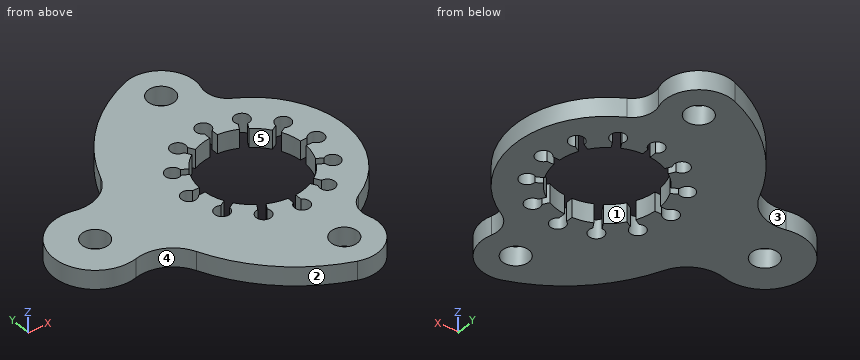
```python
from build123d import *

# Parameters (mm, degrees)
CROQUIS1_R              = 49
CROQUIS1_R_2            = 7
SALIENTE_EXTRUIR1_DEPTH = 10


with BuildPart() as part:
    # Croquis1 → Saliente-Extruir1 (new body)
    # profile 1 of 3: a face of its own
    with BuildSketch(Plane.XY):
        Circle(CROQUIS1_R)
        with BuildLine():
            ThreePointArc((11.73086121, 24.318447633), (6.988114218, 26.07999731), (2, 26.925824036))
            Line((2, 26.925824036), (2, 30.535898385))
            ThreePointArc((2, 30.535898385), (0, 38), (-2, 30.535898385))
            Line((-2, 30.535898385), (-2, 26.925824036))
            ThreePointArc((-2, 26.925824036), (-6.988114218, 26.07999731), (-11.73086121, 24.318447633))
            Line((-11.73086121, 24.318447633), (-13.535898385, 27.444863729))
            ThreePointArc((-13.535898385, 27.444863729), (-19, 32.908965344), (-17, 25.444863729))
            Line((-17, 25.444863729), (-15.194962825, 22.318447633))
            ThreePointArc((-15.194962825, 22.318447633), (-19.091883092, 19.091883092), (-22.318447633, 15.194962825))
            Line((-22.318447633, 15.194962825), (-25.444863729, 17))
            ThreePointArc((-25.444863729, 17), (-32.908965344, 19), (-27.444863729, 13.535898385))
            Line((-27.444863729, 13.535898385), (-24.318447633, 11.73086121))
            ThreePointArc((-24.318447633, 11.73086121), (-26.07999731, 6.988114218), (-26.925824036, 2))
            Line((-26.925824036, 2), (-30.535898385, 2))
            ThreePointArc((-30.535898385, 2), (-38, 0), (-30.535898385, -2))
            Line((-30.535898385, -2), (-26.925824036, -2))
            ThreePointArc((-26.925824036, -2), (-26.07999731, -6.988114218), (-24.318447633, -11.73086121))
            Line((-24.318447633, -11.73086121), (-27.444863729, -13.535898385))
            ThreePointArc((-27.444863729, -13.535898385), (-32.908965344, -19), (-25.444863729, -17))
            Line((-25.444863729, -17), (-22.318447633, -15.194962825))
            ThreePointArc((-22.318447633, -15.194962825), (-19.091883092, -19.091883092), (-15.194962825, -22.318447633))
            Line((-15.194962825, -22.318447633), (-17, -25.444863729))
            ThreePointArc((-17, -25.444863729), (-19, -32.908965344), (-13.535898385, -27.444863729))
            Line((-13.535898385, -27.444863729), (-11.73086121, -24.318447633))
            ThreePointArc((-11.73086121, -24.318447633), (-6.988114218, -26.07999731), (-2, -26.925824036))
            Line((-2, -26.925824036), (-2, -30.535898385))
            ThreePointArc((-2, -30.535898385), (0, -38), (2, -30.535898385))
            Line((2, -30.535898385), (2, -26.925824036))
            ThreePointArc((2, -26.925824036), (6.988114218, -26.07999731), (11.73086121, -24.318447633))
            Line((11.73086121, -24.318447633), (13.535898385, -27.444863729))
            ThreePointArc((13.535898385, -27.444863729), (19, -32.908965344), (17, -25.444863729))
            Line((17, -25.444863729), (15.194962825, -22.318447633))
            ThreePointArc((15.194962825, -22.318447633), (19.091883092, -19.091883092), (22.318447633, -15.194962825))
            Line((22.318447633, -15.194962825), (25.444863729, -17))
            ThreePointArc((25.444863729, -17), (32.908965344, -19), (27.444863729, -13.535898385))
            Line((27.444863729, -13.535898385), (24.318447633, -11.73086121))
            ThreePointArc((24.318447633, -11.73086121), (26.07999731, -6.988114218), (26.925824036, -2))
            Line((26.925824036, -2), (30.535898385, -2))
            ThreePointArc((30.535898385, -2), (38, 0), (30.535898385, 2))
            Line((30.535898385, 2), (26.925824036, 2))
            ThreePointArc((26.925824036, 2), (26.07999731, 6.988114218), (24.318447633, 11.73086121))
            Line((24.318447633, 11.73086121), (27.444863729, 13.535898385))
            ThreePointArc((27.444863729, 13.535898385), (32.908965344, 19), (25.444863729, 17))
            Line((25.444863729, 17), (22.318447633, 15.194962825))
            ThreePointArc((22.318447633, 15.194962825), (19.091883092, 19.091883092), (15.194962825, 22.318447633))
            Line((15.194962825, 22.318447633), (17, 25.444863729))
            ThreePointArc((17, 25.444863729), (19, 32.908965344), (13.535898385, 27.444863729))
            Line((13.535898385, 27.444863729), (11.73086121, 24.318447633))
        make_face(mode=Mode.SUBTRACT)
    # profile 2 of 3: a face of its own
    with BuildSketch(Plane.XY):
        with BuildLine():
            ThreePointArc((22.960111456, -43.287795993), (-49, 0), (22.960111456, 43.287795993))
            ThreePointArc((22.960111456, 43.287795993), (17.471680778, 49.356927241), (17.149797537, 57.533333333))
            ThreePointArc((17.149797537, 57.533333333), (12.479188654, 75.97188693), (-6.126315717, 79.925373134))
            ThreePointArc((-6.126315717, 79.925373134), (-35.730309716, 61.63434209), (-55.523644659, 33.012983471))
            ThreePointArc((-55.523644659, 33.012983471), (-62.196491498, 0), (-55.523644659, -33.012983471))
            ThreePointArc((-55.523644659, -33.012983471), (-35.730309716, -61.63434209), (-6.126315717, -79.925373134))
            ThreePointArc((-6.126315717, -79.925373134), (12.479188654, -75.97188693), (17.149797537, -57.533333333))
            ThreePointArc((17.149797537, -57.533333333), (17.471680778, -49.356927241), (22.960111456, -43.287795993))
        make_face()
        with Locations((0, -63)):
            Circle(CROQUIS1_R_2, mode=Mode.SUBTRACT)
        with Locations((0, 63)):
            Circle(CROQUIS1_R_2, mode=Mode.SUBTRACT)
    # profile 3 of 3: a face of its own
    with BuildSketch(Plane.XY):
        with BuildLine():
            ThreePointArc((-55.523644659, -33.012983471), (-62.196491498, 0), (-55.523644659, 33.012983471))
            ThreePointArc((-55.523644659, 33.012983471), (-64.981782963, 22.905981014), (-78.737580645, 21.361342246))
            ThreePointArc((-78.737580645, 21.361342246), (-106, 0), (-78.737580645, -21.361342246))
            ThreePointArc((-78.737580645, -21.361342246), (-64.981782963, -22.905981014), (-55.523644659, -33.012983471))
        make_face()
        with Locations((-84, 0)):
            Circle(CROQUIS1_R_2, mode=Mode.SUBTRACT)
    extrude(amount=SALIENTE_EXTRUIR1_DEPTH)


solid = part.part
```
Check sheet for the modelled part. Datum: model origin and axes. Units: mm. Face numbers are marked on the shaded views. A direction names the side the tool comes from. Round coordinates to 2 decimals unless told otherwise and drop trailing zeros. Order: outer loops, then holes, each group sorted by start corner. A loop starts at its lowest first (then second) coordinate and runs counter-clockwise, first axis right, second up. Notation, with made-up numbers: (42.5, 56.5) - (82.5, 56.5) arc R9 ccw to (82.5, 73.5) - close; hole circle Ø6 at (20.25, -38). An arc over 180 degrees is marked (long way). Write item = value, one per line.
Q1. Section check B-B (y = -63). Record the boundary of the cut face in (x, z), and give its area (3 significant figures).
Computed:
outline = (-34.26, 0) - (-7, 0) - (-7, 10) - (-34.26, 10) - close; (7, 0) - (18, 0) - (18, 10) - (7, 10) - close
area = 383 mm^2
Q2. Section check D-D (z = 3.75). State how many separate pieces and enclosed holes the cut face has, and give its area (3 significant figures).
Computed:
separate_pieces = 1
enclosed_holes = 4
area = 10,600 mm^2
Q3. Go/stop test with flat-tipped pins: pin 1 (4 mm diameter, centred on y = -29, z = 7, fed in from -X); pin 2 (6 mm diameter, centred on x = -22, z = 4, fed in from -Y); pin 3 (4 mm diameter, centred on x = -28, z = 3.5, fed in from -Y); pin 4 (9 mm diameter, centred on x = 34, y = 0, fed in from -Z). Record where each tip stops, or that it passes through.
Computed:
pin_1 = -59.46
pin_2 = -74.01
pin_3 = -69.59
pin_4 = 0
Q4. Section check C-C (x = -84). Record the boundary of the cut face in (y, z).
Computed:
outline = (-22, 0) - (-7, 0) - (-7, 10) - (-22, 10) - close; (7, 0) - (22, 0) - (22, 10) - (7, 10) - close
Q5. Draft check along Y on the marked faces 3, 4 and 5. Enter one of: pulls with the +Y half, pulls with the -Y half, needs draft (parallel to the pull), parting line crosses it, or undercut.
Computed:
face_3 = pulls with the +Y half
face_4 = pulls with the -Y half
face_5 = undercut
Q6. Tool access check on the marked faces 1 and 2. Record the directions out of +Z, -Z, +X, -X, +Y, -Y that give a thin tool (end or side, any length) a straight path to the whole face; none if there is none.
Computed:
face_1 = +Z, -Z
face_2 = +Z, -Z, -X, -Y
Q7. Thickness scan on line 1 along X through (y, z) = (3, 0.5); line 2 along Y through (x, z) = (-17, 7.25); line 3 along X through (y, z) = (17.5, 8.5). Record the ranges inside material, lowest first.
Computed:
line_1 = -105.79 to -90.32, -77.68 to -36.65, -31.35 to -26.83, 26.83 to 31.35, 36.65 to 48.91
line_2 = -75.1 to -33.44, -25.44 to -20.98, 20.98 to 25.44, 33.44 to 75.1
line_3 = -97.33 to -33.41, -25.48 to -20.56, 20.56 to 25.48, 33.41 to 45.77
Q8. Section check A-A (x = 0). Record the boundary of the cut face in (y, z).
Computed:
outline = (-81, 0) - (-70, 0) - (-70, 10) - (-81, 10) - close; (-56, 0) - (-38, 0) - (-38, 10) - (-56, 10) - close; (38, 0) - (56, 0) - (56, 10) - (38, 10) - close; (70, 0) - (81, 0) - (81, 10) - (70, 10) - close
